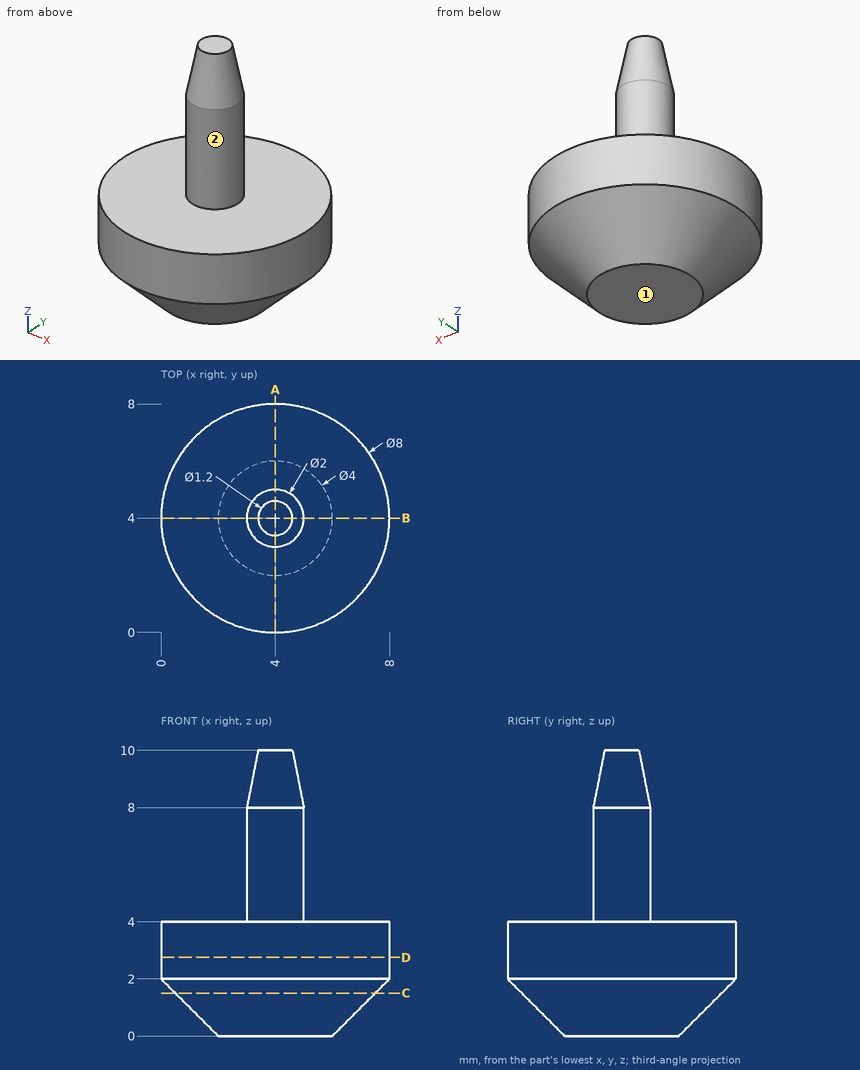
Here's the drawing with two shaded views (mm, measured from the low corner). I have some questions. A direction names the side the tool comes from. Coordinates: 2 decimals unless noted, no trailing zeros. Write each loop counter-clockwise with the first axis right and the second up, starting at its lowest first coordinate (ties: lowest second). Pieces come first, ordered by that corner, then holes. Notation, with made-up numbers: M 1.25,-11.75 L 47.25,-11.75 A20 cw 47.25,15.25 Z; hole C 77,-14.5 d6. An arc over 180 degrees is marked long. Answer as CSV lines item,"result".
Item 1: I'm going to push a flat-ended pin straight in: P1, Ø2, axis at y = 2, z = 1.5, coming from the -X side. Where does the tip first touch, or does it pass through?
Geometry results:
P1,"stops at x = 0.16"
Item 2: Imagine slicing it at D-D on z = 2.75. List the corners of the cut face in (x, y) for me.
Geometry results:
outline,"C 4,4 d8"
Item 3: Please list where these lines run through material, in increasing order: line 1 along Z through (x, y) = (2.75, 3.5); line 2 along X through (y, z) = (2, 3.5); line 3 along X through (y, z) = (1.75, 2.25).
Geometry results:
line 1,"z = 0 to 4"
line 2,"x = 0.54 to 7.46"
line 3,"x = 0.69 to 7.31"
Item 4: Imagine slicing it at C-C on z = 1.5. List the corners of the cut face in (x, y) for me.
Geometry results:
outline,"C 4,4 d7"
Item 5: Imagine slicing it at A-A on x = 4. List the corners of the cut face in (y, z) for me.
Geometry results:
outline,"M 0,2 L 2,0 L 6,0 L 8,2 L 8,4 L 5,4 L 5,8 L 4.6,10 L 3.4,10 L 3,8 L 3,4 L 0,4 Z"
Item 6: On a 3-axis mill with a long thin cutter (end or side, diameter ignored), from which of +Z, -Z, +X, -X, +Y, -Y can I reach the whole of each face in a straight line? I mean the marked faces 1 and 2. Say none if no direction works.
Geometry results:
face 1,"-Z, +X, -X, +Y, -Y"
face 2,"+Z"
